Could you check a few things on this model? Use its own coordinates, in mm. Face numbers are marked on the shaded views. A direction names the side the tool comes from. Give positions to 0.01 mm unless a question says otherwise; leave off trailing zeros. Order: outer loops, then holes, each group sorted by start corner. A loop starts at its lowest first (then second) coordinate and runs counter-clockwise, first axis right, second up.
(1) Imagine slicing it at C-C, the plane z = 9.5. Write out the boundary of the cut face in (x, y).
(2) Imagine slicing it at B-B, the plane y = 9. Write out the boundary of the cut face in (x, z).
(3) Imagine slicing it at A-A, the plane x = -0.25. Write out the boundary of the cut face in (y, z).
(4) On a 3-axis mill with a long thin cutter (end or side, diameter ignored), from which of +Z, -Z, +X, -X, +Y, -Y can I reach the whole of each face in a straight line? I mean the marked faces 1, 2 and 3. Say none if no direction works.
(5) If I drill on probe 1 along Z at (x, y) = (2.75, -4); probe 2 along Z at (x, y) = (2, 61.5); probe 3 along Y at (x, z) = (-2.5, 9), over which ranges is the centre line in solid material (lowest first)?
(6) Will this pin go through, and if not, where does the flat tip stop? pin 1 (5 mm diameter, centred on x = -0.5, y = 4.5, fed in from +Z).
(7) Imagine slicing it at D-D, the plane y = 59. Write out the boundary of the cut face in (x, z), then the cut area to 3 significant figures.
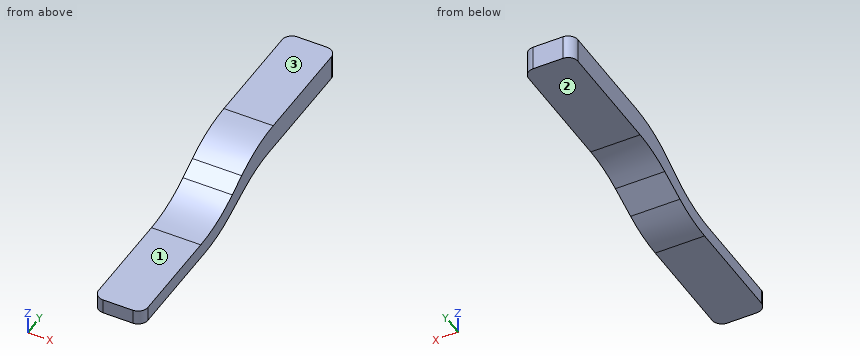
from build123d import *

# Parameters (mm, degrees)
F0_W     = 30
F0_H     = 5
F1_DEPTH = 5
F2_R     = 25
F3_R     = 2


# Not quite as in the source:
# - a feature names something its author has since deleted; it is built from what else it names


with BuildPart() as f1:
    # F0 (on Right) → F1 (new body, symmetric)
    with BuildSketch(Plane.YZ):
        Polygon((-8, 0), (0, 0), (20, 0), (20, 3), (0, 3), (-8, 3), align=None)
        Polygon((20, 3), (20, 0), (34.5558710396, 5.7734296471), (34.5558710396, 10.7734296471), align=None)
        with Locations((49.5558710396, 8.2734296471)):
            Rectangle(F0_W, F0_H)
    extrude(amount=F1_DEPTH, both=True)

    # F2
    f2_edges = [f1.edges().sort_by_distance(p)[0] for p in [
        (0, 20, 3),
        (0, 34.555871, 10.77343),
        (0, 34.555871, 5.77343),
        (0, 20, 0),
    ]]
    fillet(f2_edges, radius=F2_R)

    # F3
    f3_edges = [f1.edges().sort_by_distance(p)[0] for p in [
        (5, 64.555871, 8.27343),
        (-5, 64.555871, 8.27343),
        (5, -8, 1.5),
        (-5, -8, 1.5),
    ]]
    fillet(f3_edges, radius=F3_R)


solid = f1.part
Answer block:
1. outline: (-5, 32.94) - (5, 32.94) - (5, 62.56) arc R2 ccw to (3, 64.56) - (-3, 64.56) arc R2 ccw to (-5, 62.56) - close
2. outline: (-5, 0) - (5, 0) - (5, 3) - (-5, 3) - close
3. outline: (-8, 0) - (15.22, 0) arc R25 ccw to (24.44, 1.76) - (30.12, 4.01) arc R25 cw to (39.33, 5.77) - (64.56, 5.77) - (64.56, 10.77) - (40.81, 10.77) arc R25 ccw to (29.04, 7.83) - (25.52, 5.95) arc R25 cw to (13.74, 3) - (-8, 3) - close
4. face 1: +Z, +X, -X, -Y
4. face 2: -Z, +X, -X, +Y
4. face 3: +Z, +X, -X, +Y, -Y
5. probe 1: z = 0 to 3
5. probe 2: z = 5.77 to 10.77
5. probe 3: y = 31.57 to 64.56
6. pin 1: stops at z = 3
7. outline: (-5, 5.77) - (5, 5.77) - (5, 10.77) - (-5, 10.77) - close
7. area: 50.0 mm2
